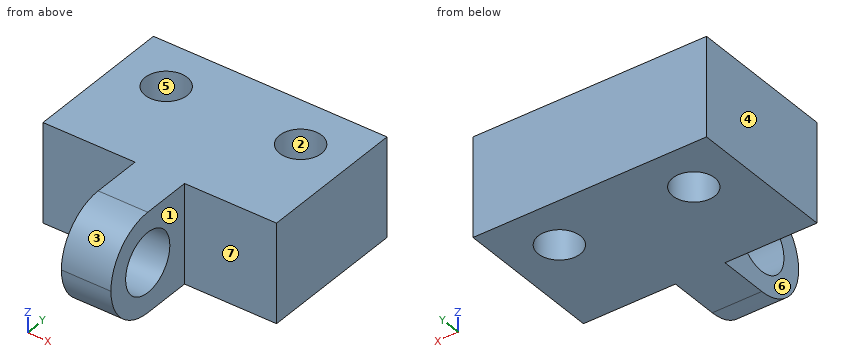
```python
from build123d import *

# Parameters (mm, degrees)
EXTRUDE1_DEPTH                 = 20
F_12_0_12_DIAMETER_HOLE1_D     = 12
F_12_0_12_DIAMETER_HOLE1_DEPTH = 47.13
F_12_0_12_DIAMETER_HOLE1_TIP   = 3.605163714
F_8_5_8_5_DIAMETER_HOLE2_D     = 8.5
FILLET1_R                      = 10


with BuildPart() as part:
    # Sketch1 → Extrude1 (new body)
    with BuildSketch(Plane.XY):
        Polygon((0, 12.157460585), (18.564852768, 12.157460585), (18.564852768, -7.842539415), (28.564852768, -7.842539415), (28.564852768, 12.157460585), (47.129705535, 12.157460585), (47.129705535, 42.157460585), (0, 42.157460585), align=None)
    extrude(amount=EXTRUDE1_DEPTH)

    # Ø12.0 (12) Diameter Hole1
    with Locations(Plane(origin=(47.129705535, 2.157460585, 10), x_dir=(0, 0, 1), z_dir=(1, 0, 0))):
        with Locations((0, 0)):
            Hole(F_12_0_12_DIAMETER_HOLE1_D / 2, depth=F_12_0_12_DIAMETER_HOLE1_DEPTH)
            with Locations((0, 0, -(F_12_0_12_DIAMETER_HOLE1_DEPTH + F_12_0_12_DIAMETER_HOLE1_TIP / 2))):  # 118° drill point
                Cone(0, F_12_0_12_DIAMETER_HOLE1_D / 2, F_12_0_12_DIAMETER_HOLE1_TIP, mode=Mode.SUBTRACT)

    # Ø8.5 (8.5) Diameter Hole2 (through all)
    with Locations(Plane(origin=(37.129705535, 32.157460585, 20), x_dir=(1, 0, 0), z_dir=(0, 0, 1))):
        with Locations((0, 0), (-27.129705535, 0)):
            Hole(F_8_5_8_5_DIAMETER_HOLE2_D / 2)

    # Fillet1
    fillet1_edges = [part.edges().sort_by_distance(p)[0] for p in [
        (23.564852768, -7.842539415, 20),
        (23.564852768, -7.842539415, 0),
    ]]
    fillet(fillet1_edges, radius=FILLET1_R - 0.0001)  # a hair under: the kernel refuses the full size


solid = part.part
```
Could you check a few things on this model? Use its own coordinates, in mm. Face numbers are marked on the shaded views. A direction names the side the tool comes from. Give positions to 0.01 mm unless a question says otherwise; leave off trailing zeros. Write each loop counter-clockwise with the first axis right and the second up, starting at its lowest first coordinate (ties: lowest second). Pieces come first, ordered by that corner, then holes. Notation, with made-up numbers: (-3.5, 81.5) -> (4.5, 81.5) arc R20 ccw to (4.5, 97.5) -> close; hole circle Ø1 at (-10.75, 2.25). An arc over 180 degrees is marked (long way). Write each question's results on one line, items separated by ' | '.
1. I want a section at D-D, the plane z = 17.5. Write out the boundary of the cut face in (x, y), then the cut area to 3 significant figures.
Check sheet entries:
outline: (0, 12.16) -> (18.56, 12.16) -> (18.56, -4.46) -> (28.56, -4.46) -> (28.56, 12.16) -> (47.13, 12.16) -> (47.13, 42.16) -> (0, 42.16) -> close; hole circle Ø8.5 at (10, 32.16); hole circle Ø8.5 at (37.13, 32.16) | area: 1,470 mm²
2. I need wall thicknesses on L1, parallel to X at y = 32.5, z = 14.75; L2, parallel to Y at x = 37, z = 15.25; L3, parallel to Y at x = 24.25, z = 10. Which ranges of each line are inside material? Lowest first, please.
Check sheet entries:
L1: x = 0 to 5.76, 14.24 to 32.89, 41.37 to 47.13 | L2: y = 12.16 to 27.91, 36.41 to 42.16 | L3: y = -7.84 to -3.84, 8.16 to 42.16
3. On a 3-axis mill with a long thin cutter (end or side, diameter ignored), from which of +Z, -Z, +X, -X, +Y, -Y can I reach the whole of each face in a straight line? I mean the marked faces 5, 6 and 7. Say none if no direction works.
Check sheet entries:
face 5: +Z, -Z | face 6: +Z, -Z, -X, -Y | face 7: +Z, -Z, +X, -Y
4. I want a section at B-B, the plane z = 13.5. Write out the boundary of the cut face in (x, y), then the cut area to 3 significant figures.
Check sheet entries:
outline: (0, 12.16) -> (18.56, 12.16) -> (18.56, 7.03) -> (28.56, 7.03) -> (28.56, 12.16) -> (47.13, 12.16) -> (47.13, 42.16) -> (0, 42.16) -> close; (18.56, -7.21) -> (28.56, -7.21) -> (28.56, -2.72) -> (18.56, -2.72) -> close; hole circle Ø8.5 at (10, 32.16); hole circle Ø8.5 at (37.13, 32.16) | area: 1,400 mm²
5. I want a section at A-A, the plane x = 10. Write out the boundary of the cut face in (y, z).
Check sheet entries:
outline: (12.16, 0) -> (27.91, 0) -> (27.91, 20) -> (12.16, 20) -> close; (36.41, 0) -> (42.16, 0) -> (42.16, 20) -> (36.41, 20) -> close
6. If we mould it in two halves opening along X, with no side actions, what happens to the marked faces 1, 2, 3 and 4? For each: released by +X, released by -X, zero draft, split by the parting line, or undercut.
Check sheet entries:
face 1: released by +X | face 2: undercut | face 3: zero draft | face 4: released by -X
7. Will these pins go through, and if not, where does the flat tip stop? pin 1 Ø5 at (x, y) = (37.13, 32.16) entering from +Z; pin 2 Ø3 at (x, z) = (15, 11) entering from -Y; pin 3 Ø6 at (x, z) = (20, 15.5) entering from -Y (3 decimals); pin 4 Ø6 at (y, z) = (2.5, 6) entering from -X.
Check sheet entries:
pin 1: passes through | pin 2: stops at y = 12.16 | pin 3: stops at y = -7.525 | pin 4: stops at x = 18.56
8. I want a section at C-C, the plane y = 5.5. Write out the boundary of the cut face in (x, z).
Check sheet entries:
outline: (18.56, 0) -> (28.56, 0) -> (28.56, 5.02) -> (18.56, 5.02) -> close; (18.56, 14.98) -> (28.56, 14.98) -> (28.56, 20) -> (18.56, 20) -> close
